Autodesk Inventor part; units mm, degrees
ref_plane "YZ Plane" through (0, 0, 0) normal (1, 0, 0) x (0, 1, 0)
ref_plane "XZ Plane" through (0, 0, 0) normal (0, 1, 0) x (-1, 0, 0)
ref_plane "XY Plane" through (0, 0, 0) normal (0, 0, 1) x (1, 0, 0)
sketch "草图1" plane through (0, 0, 0) normal (0, 0, 1) x (1, 0, 0)
  line L0 (0, 0) -> (32.5, 0)
  line L1 (32.5, 0) -> (32.5, 60)
  line L2 (32.5, 60) -> (40, 60)
  line L3 (40, 60) -> (40, 80)
  line L4 (40, 80) -> (0, 80)
  line L5 (0, 80) -> (0, 0)
  dimension "d0" = 32.5
  dimension "d1" = 60
  dimension "d2" = 7.5
  dimension "d3" = 20
revolve "旋转1" add sketch "草图1" angle 360 about axis through (0, 80, 0) along (0, -1, 0)
sketch "草图2" plane through (0, 80, 0) normal (0, 1, 0) x (1, 0, 0)
  circle A0 centre (0, 0) radius 40
hole "孔1" at (0, 80, 0) direction (0, -1, 0) diameter 45.6699 end through all
chamfer "倒角1" distance 2 angle 45 1 edges at (0, 0, -22.8349)
sketch "草图3" plane through (0, 80, 0) normal (0, 1, 0) x (1, 0, 0)
  circle A0 centre (0, 0) radius 40
  point P0 (40, 0)
hole "孔2" at (40, 80, 0) direction (0, -1, 0) diameter 8.376 depth 17
properties part number "螺套"
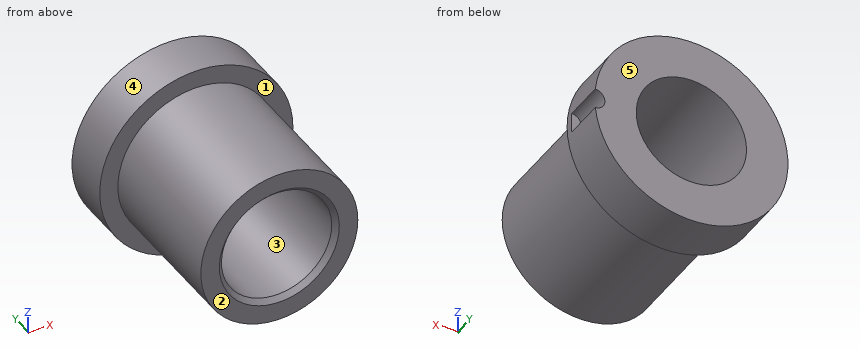
Design review of the part built by this model. Coordinates are the model's own, in mm. Face numbers are marked on the shaded views. A direction names the side the tool comes from. Coordinates: 2 decimals unless noted, no trailing zeros. Order: outer loops, then holes, each group sorted by start corner. A loop starts at its lowest first (then second) coordinate and runs counter-clockwise, first axis right, second up. Notation, with made-up numbers: (-8.75, 16.5) -> (8.25, 16.5) arc R29 cw to (8.25, 41.5) -> close; hole circle Ø4 at (69.25, -12.5). An arc over 180 degrees is marked (long way). One line per item, written item: value. Start each with the question number.
Q1. Mouldability with a two-part tool opening along X and no side actions: class the marked faces 3, 4 and 5 as pulls with the +X half, pulls with the -X half, needs draft (parallel to the pull), parting line crosses it, or undercut.
Q2. For probe 1 along Z at (x, y) = (0, 40); probe 2 along Y at (x, z) = (12, 33); probe 3 along Z at (x, y) = (12, 72), list the stretches that pass through material, from the lowest coordinate up.
Q3. Take a section at D-D, the plane x = -29. State the section outline as (y, z) points.
Q4. Take a section at C-C, the plane y = 35. State the section outline as (x, z) points, then the cut area to 3 significant figures.
Q5. Take a section at B-B, the plane x = 0. State the section outline as (y, z) points, then the cut area to 3 significant figures.
Q6. Take a section at A-A, the plane z = 0. State the section outline as (x, y) points, then the cut area to 3 significant figures.
Q7. Tool access review of the marked faces 1 and 2: name each direction out of +Z, -Z, +X, -X, +Y, -Y from which nothing blocks a thin tool from reaching the whole face with its end or side.
Q8. Insertion check: pin 1 Ø1.5 at (y, z) = (53, 16.5) entering from -X; pin 2 Ø5 at (y, z) = (38, -25.5) entering from +X; pin 3 Ø4 at (y, z) = (12.5, 25) entering from -X. Each pin has a flat end and moves straight along its axis. Give the tip position at first contact, or say it passes through.
Values follow:
1. face 3: undercut
1. face 4: parting line crosses it
1. face 5: needs draft
2. probe 1: z = -32.5 to -22.83, 22.83 to 32.5
2. probe 2: y = 60 to 80
2. probe 3: z = -38.16 to -19.43, 19.43 to 38.16
3. outline: (0, -14.67) -> (60, -14.67) -> (60, -27.55) -> (80, -27.55) -> (80, 27.55) -> (60, 27.55) -> (60, 14.67) -> (0, 14.67) -> close
4. outline: circle Ø65 at (0, 0); hole circle Ø45.67 at (0, 0)
4. area: 1,680 mm2
5. outline: (0, -32.5) -> (60, -32.5) -> (60, -40) -> (80, -40) -> (80, -22.83) -> (2, -22.83) -> (0, -24.83) -> close; (0, 24.83) -> (2, 22.83) -> (80, 22.83) -> (80, 40) -> (60, 40) -> (60, 32.5) -> (0, 32.5) -> close
5. area: 1,840 mm2
6. outline: (-40, 60) -> (-32.5, 60) -> (-32.5, 0) -> (-24.83, 0) -> (-22.83, 2) -> (-22.83, 80) -> (-40, 80) -> close; (22.83, 2) -> (24.83, 0) -> (32.5, 0) -> (32.5, 60) -> (40, 60) -> (40, 63) -> (35.81, 63) -> (35.81, 80) -> (22.83, 80) -> close
6. area: 1,770 mm2
7. face 1: -Y
7. face 2: +Z, -Z, +X, -X, -Y
8. pin 1: stops at x = -28.43
8. pin 2: stops at x = 22.96
8. pin 3: stops at x = -22.96
